For this review, take the finished solid that the model builds, in its own axes (mm). A direction names the side the tool comes from. Round coordinates to 2 decimals unless told otherwise and drop trailing zeros. Loops run counter-clockwise (first coordinate to the right, second up) from the corner with the lowest first, then second, coordinate; pieces in that order, holes last. Notation, with made-up numbers: (54, -34.75) -> (66, -34.75) arc R18 cw to (66, -24.75) -> close; hole circle Ø3 at (39, 71). An arc over 180 degrees is marked (long way). Write each question's results on one line, items separated by ' | '.
```python
from build123d import *

# Parameters (mm, degrees)
SKETCH2_R           = 7.5
SKETCH2_R_2         = 5
SKETCH2_W           = 6.35
SKETCH2_H           = 6.35
BOSS_EXTRUDE1_DEPTH = 10
SKETCH2_4_R         = 5
BOSS_EXTRUDE2_DEPTH = 20
SKETCH2_5_R         = 7.5
SKETCH2_5_R_2       = 5
BOSS_EXTRUDE3_DEPTH = 3
SKETCH3_R           = 2
CUT_EXTRUDE1_DEPTH  = 8.5


with BuildPart() as part:
    # Sketch2 → Boss-Extrude1 (new body)
    with BuildSketch(Plane(origin=(0, 0, 0), x_dir=(1, 0, 0), z_dir=(0, 1, 0))):
        with Locations(Location((0, 0, 0), (0, 0, 270))):
            Circle(SKETCH2_R)
        Circle(SKETCH2_R_2, mode=Mode.SUBTRACT)
        Circle(SKETCH2_R_2)
        Rectangle(SKETCH2_W, SKETCH2_H, mode=Mode.SUBTRACT)
    extrude(amount=BOSS_EXTRUDE1_DEPTH)

    # Sketch2<4> → Boss-Extrude2 (add)
    with BuildSketch(Plane(origin=(0, 0, 0), x_dir=(1, 0, 0), z_dir=(0, 1, 0))):
        with Locations(Location((0, 0, 0), (0, 0, 270))):
            Circle(SKETCH2_4_R)
    extrude(amount=-BOSS_EXTRUDE2_DEPTH)

    # Sketch2<5> → Boss-Extrude3 (add)
    with BuildSketch(Plane(origin=(0, 0, 0), x_dir=(1, 0, 0), z_dir=(0, 1, 0))):
        with Locations(Location((0, 0, 0), (0, 0, 270))):
            Circle(SKETCH2_5_R)
        with Locations(Location((0, 0, 0), (0, 0, 270))):
            Circle(SKETCH2_5_R_2, mode=Mode.SUBTRACT)
    extrude(amount=-BOSS_EXTRUDE3_DEPTH)

    # Sketch3 → Cut-Extrude1 (cut)
    with BuildSketch(Plane.XZ.offset(20)):
        with Locations(Location((0, 0, 0), (0, 0, 270))):
            Circle(SKETCH3_R)
    extrude(amount=-CUT_EXTRUDE1_DEPTH, mode=Mode.SUBTRACT)


solid = part.part
```
1. Consider section B-B (y = 1). State the section outline as (x, z) points (3 decimals), plus the area to 3 significant figures.
Values found:
outline: circle Ø15 at (0, 0); hole (-3.175, -3.175) -> (3.175, -3.175) -> (3.175, 3.175) -> (-3.175, 3.175) -> close | area: 136 mm2
2. Draft analysis for pull direction X (two halves, no side actions). For faces 4 (the face through (3.4, 10, -0.1)), 5 (the face through (-4.88, -11.38, -1.08)), 6 (the face through (0, 5, 3.175)), state which applies: released by +X, released by -X, zero draft, split by the parting line, or undercut.
Values found:
face 4: zero draft | face 5: split by the parting line | face 6: undercut
3. Consider section A-A (x = 0). State the section outline as (y, z) points (3 decimals).
Values found:
outline: (-20, -5) -> (-3, -5) -> (-3, -7.5) -> (10, -7.5) -> (10, -3.175) -> (0, -3.175) -> (0, 3.175) -> (10, 3.175) -> (10, 7.5) -> (-3, 7.5) -> (-3, 5) -> (-20, 5) -> (-20, 2) -> (-11.5, 2) -> (-11.5, -2) -> (-20, -2) -> close
4. To check wall thickness, follow probe 1 along X at (y, z) = (-14.75, 0); probe 2 along Y at (x, z) = (-4, -5.25); probe 3 along X at (y, z) = (5.5, 1.75) (3 decimals). State the ranges of each line that lie inside material, in increasing order.
Values found:
probe 1: x = -5 to -2, 2 to 5 | probe 2: y = -3 to 10 | probe 3: x = -7.293 to -3.175, 3.175 to 7.293
5. Consider section C-C (z = 0). State the section outline as (x, y) points (3 decimals).
Values found:
outline: (-7.5, -3) -> (-5, -3) -> (-5, -20) -> (-2, -20) -> (-2, -11.5) -> (2, -11.5) -> (2, -20) -> (5, -20) -> (5, -3) -> (7.5, -3) -> (7.5, 10) -> (3.175, 10) -> (3.175, 0) -> (-3.175, 0) -> (-3.175, 10) -> (-7.5, 10) -> close
6. For pin 1 (1 mm diameter, centred on x = -2, y = -11.5, fed in from +Z); pin 2 (5 mm diameter, centred on x = 0.5, z = 0, fed in from +Y); pin 3 (7 mm diameter, centred on y = 4.5, z = 0.5, fed in from -X); pin 4 (3 mm diameter, centred on x = -3, y = 6.5, fed in from -Z), all flat-tipped, find the tip position at first contact; note any pin that passes through.
Values found:
pin 1: stops at z = 4.77 | pin 2: stops at y = 0 | pin 3: stops at x = -7.5 | pin 4: stops at z = -7.35
7. Consider section D-D (y = -12.5). State the section outline as (x, z) points.
Values found:
outline: circle Ø10 at (0, 0); hole circle Ø4 at (0, 0)
8. Tool access review of faces 1 (the face through (0.1, -20, 2.2)), 2 (the face through (3.175, 5, 0)), 3 (the face through (0, -11.5, 0)): name each direction out of +Z, -Z, +X, -X, +Y, -Y from which nothing blocks a thin tool from reaching the whole face with its end or side.
Values found:
face 1: +Z, -Z, +X, -X, -Y | face 2: +Y | face 3: -Y
